from build123d import *

# Parameters (mm, degrees)
F0_W     = 647.7
F0_H     = 88.9
F0_R     = 6.35
F1_DEPTH = 88.9
F2_W     = 44.45
F2_H     = 44.45
F3_DEPTH = 101.6


with BuildPart() as f1:
    # F0 (on Front) → F1 (new body)
    with BuildSketch(Plane.XZ):
        Rectangle(F0_W, F0_H)
        with Locations((-301.625, -19.05)):
            Circle(F0_R, mode=Mode.SUBTRACT)
        with Locations((301.625, -19.05)):
            Circle(F0_R, mode=Mode.SUBTRACT)
        with Locations((-301.625, 19.05)):
            Circle(F0_R, mode=Mode.SUBTRACT)
        with Locations((-63.5, 0)):
            Circle(F0_R, mode=Mode.SUBTRACT)
        with Locations((301.625, 19.05)):
            Circle(F0_R, mode=Mode.SUBTRACT)
    extrude(amount=F1_DEPTH)

    # F2 (on face) → F3 (cut)
    with BuildSketch(Plane.XY.offset(44.45)):
        with Locations((-301.625, -22.225)):
            Rectangle(F2_W, F2_H)
        with Locations((301.625, -22.225)):
            Rectangle(F2_W, F2_H)
    extrude(amount=-F3_DEPTH, mode=Mode.SUBTRACT)


solid = f1.part
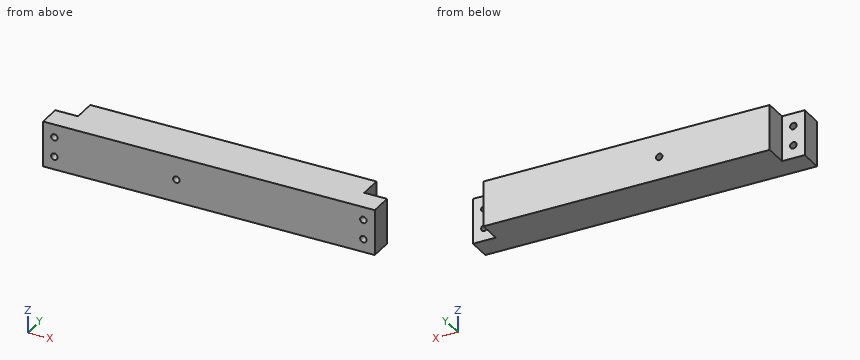
Design review of the part built by this model. Coordinates are the model's own, in mm. Give positions to 0.01 mm unless a question says otherwise; leave off trailing zeros. Order: outer loops, then holes, each group sorted by start corner. A loop starts at its lowest first (then second) coordinate and runs counter-clockwise, first axis right, second up.
1. Add section B-B, the plane y = -11. State the section outline as (x, z) points, then the cut area to 3 significant figures.
Solution:
outline: (-279.4, -44.45) - (279.4, -44.45) - (279.4, 44.45) - (-279.4, 44.45) - close; hole circle Ø12.7 at (-63.5, 0)
area: 49,600 mm2
2. Add section A-A, the plane z = 19.05. State the section outline as (x, y) points (3 decimals), then the cut area to 3 significant figures.
Solution:
outline: (-323.85, -88.9) - (-307.975, -88.9) - (-307.975, -44.45) - (-323.85, -44.45) - close; (-295.275, -88.9) - (295.275, -88.9) - (295.275, -44.45) - (279.4, -44.45) - (279.4, 0) - (-279.4, 0) - (-279.4, -44.45) - (-295.275, -44.45) - close; (307.975, -88.9) - (323.85, -88.9) - (323.85, -44.45) - (307.975, -44.45) - close
area: 52,500 mm2
3. To check wall thickness, follow L1, parallel to X at y = -62, z = -19; L2, parallel to Z at x = -63, y = -18; L3, parallel to X at y = -12.5, z = -21.5. State the ranges of each line that lie inside material, in increasing order.
Solution:
L1: x = -323.85 to -307.97, -295.28 to 295.28, 307.97 to 323.85
L2: z = -44.45 to -6.33, 6.33 to 44.45
L3: x = -279.4 to 279.4
4. Add section C-C, the plane x = -63.5. State the section outline as (y, z) points, then the cut area to 3 significant figures.
Solution:
outline: (-88.9, -44.45) - (0, -44.45) - (0, -6.35) - (-88.9, -6.35) - close; (-88.9, 6.35) - (0, 6.35) - (0, 44.45) - (-88.9, 44.45) - close
area: 6,770 mm2
5. Add section D-D, the plane z = -36. State the section outline as (x, y) points.
Solution:
outline: (-323.85, -88.9) - (323.85, -88.9) - (323.85, -44.45) - (279.4, -44.45) - (279.4, 0) - (-279.4, 0) - (-279.4, -44.45) - (-323.85, -44.45) - close
6. For pin 1 Ø22 at (x, z) = (302.5, -18) entering from +Y; pin 2 Ø2 at (y, z) = (-22.5, 24) entering from -X; pin 3 Ø22 at (y, z) = (-27, -12.5) entering from +X; pin 4 Ø14.5 at (x, z) = (-301.625, 19.05) entering from -Y, all flat-tipped, find the tip position at first contact; note any pin that passes through.
Solution:
pin 1: stops at y = -44.45
pin 2: stops at x = -279.4
pin 3: stops at x = 279.4
pin 4: stops at y = -88.9
